Here's how the part is built. I have some questions about the finished solid (model axes, mm). Face numbers are marked on the shaded views. A direction names the side the tool comes from. Give positions to 0.01 mm unless a question says otherwise; leave off trailing zeros. Order: outer loops, then holes, each group sorted by start corner. A loop starts at its lowest first (then second) coordinate and runs counter-clockwise, first axis right, second up. Notation, with made-up numbers: M -23.5,31 L 18.5,31 A11 ccw 18.5,44 Z; hole C 30,-6.5 d6. An arc over 180 degrees is marked long. Use one line per item in the form item = value.
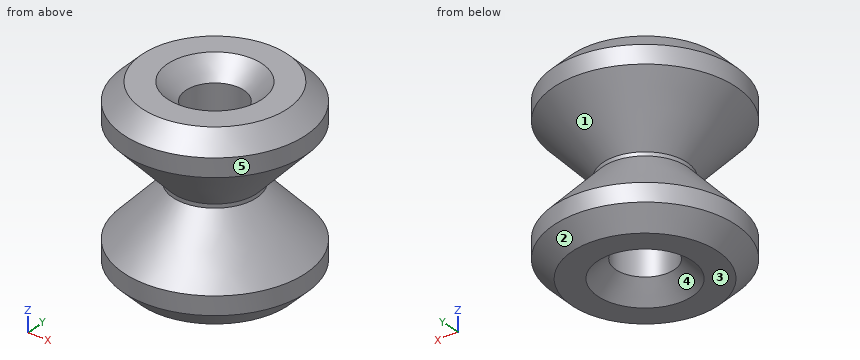
from build123d import *

# Parameters (mm, degrees)
F0_R     = 5
F0_R_2   = 1.6
F1_DEPTH = 10
F4_SIZE  = 1


with BuildPart() as f1:
    # F0 (on Top) → F1 (new body)
    with BuildSketch(Plane.XY):
        Circle(F0_R)
        Circle(F0_R_2, mode=Mode.SUBTRACT)
    extrude(amount=F1_DEPTH)

    # F2 (on Front) → F3 (revolve, cut)
    with BuildSketch(Plane.XZ):
        Polygon((5, 2), (5, 8), (2.3, 5.104604), (2.3, 4.895396), align=None)
    revolve(axis=Axis((0, 0, 10), (0, 0, 1)), mode=Mode.SUBTRACT)

    # F4
    f4_edges = [f1.edges().sort_by_distance(p)[0] for p in [
        (-5, 0, 10),
        (-5, 0, 0),
        (-1.6, 0, 10),
        (-1.6, 0, 0),
    ]]
    chamfer(f4_edges, length=F4_SIZE)


solid = f1.part
Q1. I want a section at C-C on z = 8.75. Write out the boundary of the cut face in (x, y), then the cut area to 3 significant figures.
Found:
outline = C 0,0 d10; hole C 0,0 d3.2
area = 70.5 mm²
Q2. Thinking about a two-plate mould opening in Y: for the marked faces 3, 4 and 5, which applies, +Y half, -Y half, draft (parallel to the pull), parting line (faces both ways), or undercut?
Found:
face_3 = draft
face_4 = undercut
face_5 = parting line
Q3. On a 3-axis mill with a long thin cutter (end or side, diameter ignored), from which of +Z, -Z, +X, -X, +Y, -Y can I reach the whole of each face in a straight line? I mean the marked faces 1 and 2. Say none if no direction works.
Found:
face_1 = none
face_2 = -Z
Q4. I'm going to push a flat-ended pin straight in: pin 1 Ø5 at (x, y) = (0, 0) entering from +Z. Where does the tip first touch, or does it pass through?
Found:
pin_1 = 9.9
Q5. I want a section at D-D on z = 4.5. Write out the boundary of the cut face in (x, y), then the cut area to 3 significant figures.
Found:
outline = C 0,0 d5.34; hole C 0,0 d3.2
area = 14.3 mm²
Q6. I want a section at A-A on x = 0. Write out the boundary of the cut face in (y, z).
Found:
outline = M -5,1 L -4,0 L -2.6,0 L -1.6,1 L -1.6,9 L -2.6,10 L -4,10 L -5,9 L -5,8 L -2.3,5.1 L -2.3,4.9 L -5,2 Z; M 1.6,1 L 2.6,0 L 4,0 L 5,1 L 5,2 L 2.3,4.9 L 2.3,5.1 L 5,8 L 5,9 L 4,10 L 2.6,10 L 1.6,9 Z
Q7. I need wall thicknesses on L1, parallel to Z at x = -4, y = 1; L2, parallel to Z at x = -2, y = 3; L3, parallel to X at y = -0.5, z = 4.5. Which ranges of each line are inside material? Lowest first, please.
Found:
L1 = 0.12 to 2.94, 7.06 to 9.88
L2 = 0 to 3.5, 6.5 to 10
L3 = -2.62 to -1.52, 1.52 to 2.62
